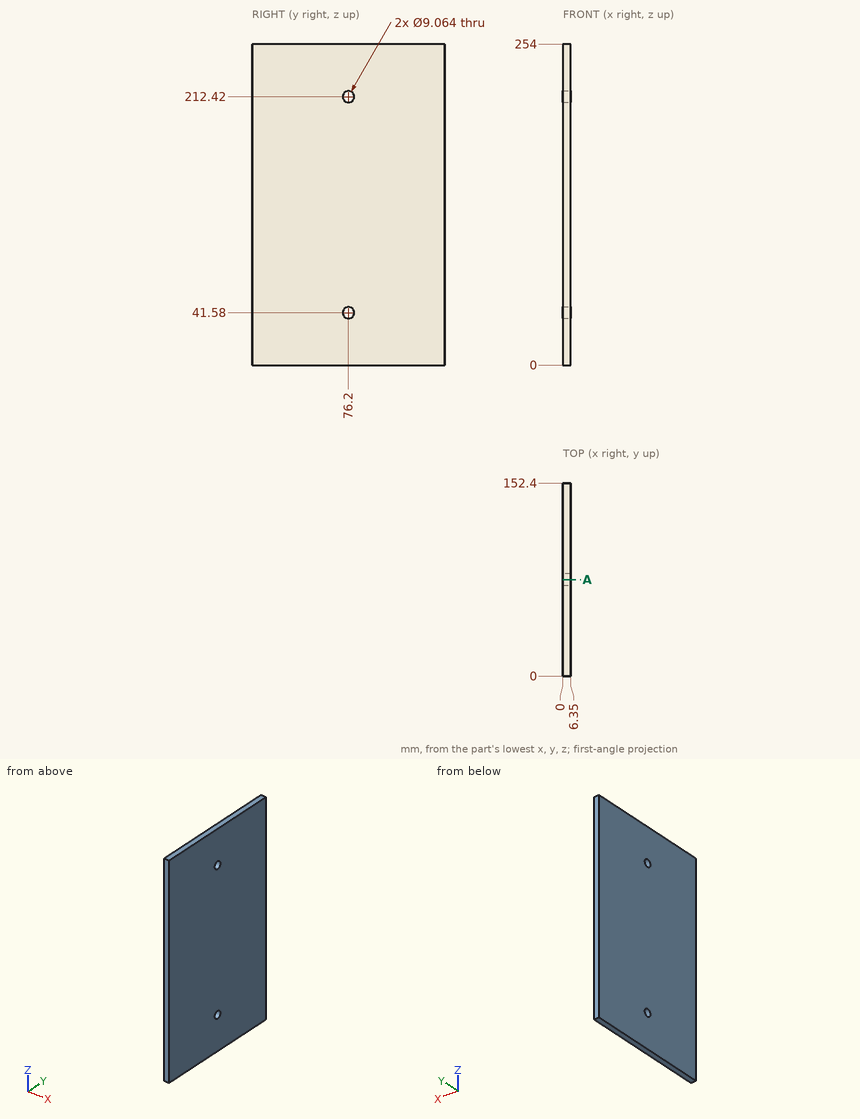
Study the drawing (mm; zero at the part's minimum x, y, z) and answer. Round coordinates to 2 decimals unless told otherwise and drop trailing zeros. Loops run counter-clockwise (first coordinate to the right, second up) from the corner with the lowest first, then second, coordinate; pieces in that order, holes last. Notation, with made-up numbers: (-14.5, 58) -> (13.5, 58) arc R25 cw to (13.5, 91) -> close; hole circle Ø6 at (-30.75, -14). An arc over 180 degrees is marked (long way). One line per item, written item: value.
1) A flat-ended cylindrical pin translates along its axis: P1, Ø10.5, axis at y = 76.2, z = 212.42, coming from the -X side. Find the tip coordinate at first contact, or state that the pin passes through.
Answer list:
P1: stops at x = 0
2) A cutting plane is placed at A-A (y = 76.2). Determine the outline of the cut face in (x, z), and give its area (3 significant figures).
Answer list:
outline: (0, 0) -> (6.35, 0) -> (6.35, 37.05) -> (0, 37.05) -> close; (0, 46.11) -> (6.35, 46.11) -> (6.35, 207.89) -> (0, 207.89) -> close; (0, 216.95) -> (6.35, 216.95) -> (6.35, 254) -> (0, 254) -> close
area: 1,500 mm²
3) Consider L1, parallel to Z at x = 1.25, y = 76.5; L2, parallel to Z at x = 2, y = 76.2; L3, parallel to Y at x = 1.5, z = 37.5 (1 decimal). Determine where each line is inside the solid, lowest interval first. Write a range as [from, to].
Answer list:
L1: z = [0, 37.06], [46.1, 207.9], [216.94, 254]
L2: z = [0, 37.05], [46.11, 207.89], [216.95, 254]
L3: y = [0, 74.2], [78.2, 152.4]
